from build123d import *

# Parameters (mm, degrees)
SKETCH2_W           = 20
SKETCH2_H           = 8
SKETCH2_R           = 1.5
BOSS_EXTRUDE3_DEPTH = 3
BOSS_EXTRUDE4_START = -12
SKETCH5_R           = 1.6
BOSS_EXTRUDE4_DEPTH = 4


with BuildPart() as part:
    # Sketch2 → Boss-Extrude3 (new body)
    with BuildSketch(Plane.XY):
        with Locations((0, 4)):
            Rectangle(SKETCH2_W, SKETCH2_H)
        with Locations((-3.25, 4.5)):
            Circle(SKETCH2_R, mode=Mode.SUBTRACT)
        with Locations(Location((3.25, 4.5, 0), (0, 0, 180))):
            Circle(SKETCH2_R, mode=Mode.SUBTRACT)
    extrude(amount=BOSS_EXTRUDE3_DEPTH)

    # Sketch5 → Boss-Extrude4 (add)
    with BuildSketch(Plane(origin=(10, 0, 0), x_dir=(0, 0, -1), z_dir=(1, 0, 0)).offset(BOSS_EXTRUDE4_START)):
        with BuildLine():
            Line((-5.5, 0), (-5.5, -8))
            ThreePointArc((-5.5, -8), (-1.5, -12), (2.5, -8))
            Line((2.5, -8), (2.5, 0))
            Line((2.5, 0), (2.5, 1))
            Line((2.5, 1), (0, 1))
            Line((0, 1), (0, 0))
            Line((0, 0), (-3, 0))
            Line((-3, 0), (-3, 1))
            Line((-3, 1), (-5.5, 1))
            Line((-5.5, 1), (-5.5, 0))
        make_face()
        with Locations(Location((-1.5, -8, 0), (0, 0, 90))):
            Circle(SKETCH5_R, mode=Mode.SUBTRACT)
    extrude(amount=BOSS_EXTRUDE4_DEPTH)


solid = part.part
Verification items for the finished model (mm, model axes). A direction names the side the tool comes from. Coordinates: 2 decimals unless noted, no trailing zeros. Loops run counter-clockwise (first coordinate to the right, second up) from the corner with the lowest first, then second, coordinate; pieces in that order, holes last. Notation, with made-up numbers: (-34.5, -26.75) -> (8.5, -26.75) arc R32 cw to (8.5, 8.25) -> close; hole circle Ø9 at (49, -16.5). An arc over 180 degrees is marked (long way). Write each question's results on one line, items separated by ' | '.
Item 1: Gauge pin test, flat ends, axial feed: pin 1 (4 mm diameter, centred on y = -7.5, z = 0.5, fed in from -X); pin 2 (3 mm diameter, centred on x = -6, y = 2.5, fed in from -Z); pin 3 (1.5 mm diameter, centred on x = -8, z = 2, fed in from -Y). Record the tip position at first contact, or that the pin passes through.
Found:
pin 1: stops at x = -2 | pin 2: stops at z = 0 | pin 3: stops at y = 0
Item 2: Tool access check on faces 1 (the face through (1.82, 4.05, 1.48)), 2 (the face through (0, 1, 4)), 3 (the face through (0, 1, -1)), 4 (the face through (6, 0, 1)), 5 (the face through (-6, 0, 1)). Record the directions out of +Z, -Z, +X, -X, +Y, -Y that give a thin tool (end or side, any length) a straight path to the whole face; none if there is none.
Found:
face 1: +Z, -Z | face 2: +Z, +X, -X, +Y | face 3: -Z, +X, -X, +Y | face 4: +Z, -Z, +X, -Y | face 5: +Z, -Z, -X, -Y
Item 3: Section check A-A, the plane z = 1.5. Enter the section's corners in (x, y).
Found:
outline: (-10, 0) -> (-2, 0) -> (-2, -6.4) -> (2, -6.4) -> (2, 0) -> (10, 0) -> (10, 8) -> (-10, 8) -> close; (-2, -12) -> (2, -12) -> (2, -9.6) -> (-2, -9.6) -> close; hole circle Ø3 at (-3.25, 4.5); hole circle Ø3 at (3.25, 4.5)
Item 4: Material ranges on L1, parallel to Z at x = -0.75, y = -8; L2, parallel to Y at x = -3.25, z = 2.3; L3, parallel to Y at x = -9, z = 1, recorded low to high.
Found:
L1: z = -2.5 to -0.1, 3.1 to 5.5 | L2: y = 0 to 3, 6 to 8 | L3: y = 0 to 8
Item 5: Mould release check, pull along X, two halves, no side actions. Record for faces 6 (the face through (0, 8, 1)), 7 (the face through (10, 4, 1)), 8 (the face through (-1.82, 4.95, 1.48)): +X half, -X half, draft (parallel to the pull), parting line (faces both ways), or undercut.
Found:
face 6: draft | face 7: +X half | face 8: undercut
Item 6: Section check D-D, the plane y = 4.5. Enter the section's corners in (x, z).
Found:
outline: (-10, 0) -> (-4.75, 0) -> (-4.75, 3) -> (-10, 3) -> close; (-1.75, 0) -> (1.75, 0) -> (1.75, 3) -> (-1.75, 3) -> close; (4.75, 0) -> (10, 0) -> (10, 3) -> (4.75, 3) -> close
Item 7: Section check B-B, the plane x = 3.25. Enter the section's corners in (y, z), plus the area to 3 significant figures.
Found:
outline: (0, 0) -> (3, 0) -> (3, 3) -> (0, 3) -> close; (6, 0) -> (8, 0) -> (8, 3) -> (6, 3) -> close | area: 15.0 mm2
Item 8: Section check C-C, the plane y = -7. Enter the section's corners in (x, z), plus the area to 3 significant figures.
Found:
outline: (-2, -2.5) -> (2, -2.5) -> (2, 0.25) -> (-2, 0.25) -> close; (-2, 2.75) -> (2, 2.75) -> (2, 5.5) -> (-2, 5.5) -> close | area: 22.0 mm2
